Solid Edge part; units mm, degrees
sketch "Sketch1" plane through (0, 0, 0) normal (0, -1, 0) x (1, 0, 0)
  line L0 (75.2427, 0) -> (0, 0)
  line L1 (0, 0) -> (-14.7573, 14.7573)
  line L2 (-14.7573, 14.7573) -> (-14.7573, 52.3)
  line L3 (-14.7573, 52.3) -> (75.2427, 52.3)
  line L4 (75.2427, 52.3) -> (75.2427, 0)
  dimension "D1" = 14.7573
extrude "Protrusion1" add sketch "Sketch1" against normal blind 2
sketch "Sketch2" plane through (30.2427, 2, 26.15) normal (0, 1, 0) x (-1, 0, 0)
  line L0 (-15, -3.65) -> (-3, -3.65)
  line L1 (-3, -3.65) -> (-3, -20.05)
  line L2 (-3, -20.05) -> (-15, -20.05)
  line L3 (-15, -20.05) -> (-15, -3.65)
  dimension "D1" = 15
  dimension "D2" = 15
extrude "Cutout1" cut sketch "Sketch2" against normal through all
sketch "Sketch3" plane through (30.2427, 2, 26.15) normal (0, 1, 0) x (-1, 0, 0)
  line L0 (-15, 0.35) -> (-3, 0.35)
  line L1 (-3, 0.35) -> (-3, 16.35)
  line L2 (-3, 16.35) -> (-15, 16.35)
  line L3 (-15, 16.35) -> (-15, 0.35)
  dimension "D1" = 3
  dimension "D2" = 15
extrude "Cutout2" cut sketch "Sketch3" against normal through all
sketch "Sketch4" plane through (30.2427, 2, 26.15) normal (0, 1, 0) x (-1, 0, 0)
  line L0 (-45, -8.15) -> (-19, -8.15)
  line L1 (-19, -8.15) -> (-19, -11.15)
  line L2 (-19, -11.15) -> (-45, -11.15)
  line L3 (-45, -11.15) -> (-45, -8.15)
  dimension "D1" = 45
  dimension "D2" = 45
extrude "Extrusionsausprägung_2" add sketch "Sketch4" along normal blind 12
sketch "Sketch5" plane through (30.2427, 2, 26.15) normal (0, 1, 0) x (-1, 0, 0)
  line L0 (-45, 26.15) -> (-21, 26.15)
  line L1 (-21, 26.15) -> (-21, 24.15)
  line L2 (-21, 24.15) -> (-45, 24.15)
  line L3 (-45, 24.15) -> (-45, 26.15)
  dimension "D1" = 45
  dimension "D2" = 21
extrude "Protrusion2" add sketch "Sketch5" along normal up to vertex (12 mm away)
sketch "Sketch6" plane through (30.2427, 2, 26.15) normal (0, 1, 0) x (-1, 0, 0)
  line L0 (30, 26.15) -> (24, 26.15)
  line L1 (24, 26.15) -> (24, 24.15)
  line L2 (24, 24.15) -> (30, 24.15)
  line L3 (30, 24.15) -> (30, 26.15)
  dimension "D1" = 30
  dimension "D2" = 30
  dimension "D3" = 30
extrude "Extrusionsausprägung_4" add sketch "Sketch6" along normal blind 7
sketch "Sketch7" plane through (30.2427, 0, 26.15) normal (0, -1, 0) x (1, 0, 0)
  circle A0 centre (-2, -16.15) radius 1
  circle A1 centre (20, -16.15) radius 1
extrude "Cutout3" cut sketch "Sketch7" against normal through all
sketch "Sketch8" plane through (30.2427, 0, 26.15) normal (0, -1, 0) x (1, 0, 0)
  circle A0 centre (33, -19.15) radius 1.3
  dimension "D1" = 33
extrude "Cutout4" cut sketch "Sketch8" against normal through all
sketch "Sketch9" plane through (30.2427, 0, 26.15) normal (0, -1, 0) x (1, 0, 0)
  circle A0 centre (-30.6, -21.15) radius 1.3
  dimension "D1" = 30.6
extrude "Cutout5" cut sketch "Sketch9" against normal through all
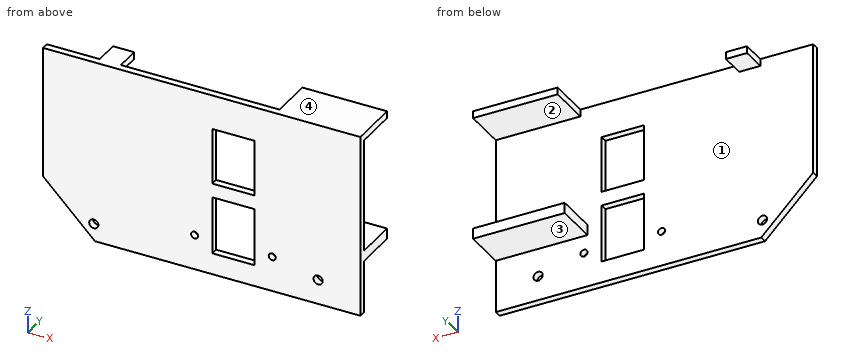
Source: CAD feature listing. Evaluate the final solid. Frame: model axes, mm. Face numbers are marked on the shaded views. Coordinates: 2 decimals unless noted, no trailing zeros. Write each loop counter-clockwise with the first axis right and the second up, starting at its lowest first coordinate (ties: lowest second). Pieces come first, ordered by that corner, then holes. Notation, with made-up numbers: M 24,35.25 L 54,35.25 A29 ccw 54,69.25 Z; hole C -17.5,28 d8. An arc over 180 degrees is marked long. Use a Markdown table: item, result.
1) Section C-C, the plane y = 7.75. Output: boundary loops of the cut face in (x, z), then the cut area to 3 significant figures.
Conclusion:
| item | result |
|---|---|
| outline | M 0.24,50.3 L 6.24,50.3 L 6.24,52.3 L 0.24,52.3 Z; M 49.24,15 L 75.24,15 L 75.24,18 L 49.24,18 Z; M 51.24,50.3 L 75.24,50.3 L 75.24,52.3 L 51.24,52.3 Z |
| area | 138 mm^2 |
2) Section B-B, the plane x = 43.5. Output: boundary loops of the cut face in (y, z), then the cut area to 3 significant figures.
Conclusion:
| item | result |
|---|---|
| outline | M 0,0 L 2,0 L 2,6.1 L 0,6.1 Z; M 0,22.5 L 2,22.5 L 2,26.5 L 0,26.5 Z; M 0,42.5 L 2,42.5 L 2,52.3 L 0,52.3 Z |
| area | 39.8 mm^2 |
3) Mould query, pull axis Z, two halves, no side actions, for the marked faces 1, 2, 3 and 4. Classes: pulls with the +Z half, pulls with the -Z half, needs draft (parallel to the pull), parting line crosses it, or undercut.
Conclusion:
| item | result |
|---|---|
| face 1 | undercut |
| face 2 | undercut |
| face 3 | pulls with the -Z half |
| face 4 | pulls with the +Z half |
4) First-contact query: pin 1 Ø3 at (x, z) = (50.24, 10) entering from +Y; pin 2 Ø1.6 at (x, z) = (4.5, 51) entering from +Y; pin 3 Ø4 at (y, z) = (5.5, 29.5) entering from +X; pin 4 Ø1 at (y, z) = (4.5, 51) entering from -X. Flat tips, straight axial feed; report the tip coordinate or a pass-through.
Conclusion:
| item | result |
|---|---|
| pin 1 | stops at y = 2 |
| pin 2 | stops at y = 9 |
| pin 3 | passes through |
| pin 4 | stops at x = 0.24 |
5) Ray query, L1, parallel to Z at x = 63, y = 12.5; L2, parallel to Y at x = 56.5, z = 6.5; L3, parallel to X at y = 6.5, z = 15.5. Return the intervals inside material, ascending.
Conclusion:
| item | result |
|---|---|
| L1 | z = 15 to 18, 50.3 to 52.3 |
| L2 | y = 0 to 2 |
| L3 | x = 49.24 to 75.24 |
6) Section A-A, the plane z = 10. Output: boundary loops of the cut face in (x, y), then the cut area to 3 significant figures.
Conclusion:
| item | result |
|---|---|
| outline | M -10,0 L 27.24,0 L 27.24,2 L -10,2 Z; M 29.24,0 L 33.24,0 L 33.24,2 L 29.24,2 Z; M 45.24,0 L 49.24,0 L 49.24,2 L 45.24,2 Z; M 51.24,0 L 75.24,0 L 75.24,2 L 51.24,2 Z |
| area | 138 mm^2 |
7) Section D-D, the plane z = 20.5. Output: boundary loops of the cut face in (x, y).
Conclusion:
| item | result |
|---|---|
| outline | M -14.76,0 L 33.24,0 L 33.24,2 L -14.76,2 Z; M 45.24,0 L 75.24,0 L 75.24,2 L 45.24,2 Z |
